```python
from build123d import *

# Parameters (mm, degrees)
F1_DEPTH       = 5
F2_W           = 15
F2_H           = 5
F3_DEPTH       = 10
F4_R           = 5
F6_D           = 4.2
F6_CSINK_D     = 8.96
F6_CSINK_ANGLE = 90


with BuildPart() as f1:
    # F0 (on Top) → F1 (new body)
    with BuildSketch(Plane.XY):
        with BuildLine():
            Line((29.5, 20), (-29.5, 20))
            ThreePointArc((-29.5, 20), (-31.62132, 19.12132), (-32.5, 17))
            Line((-32.5, 17), (-32.5, -2.5))
            ThreePointArc((-32.5, -2.5), (-31.767767, -4.267767), (-30, -5))
            ThreePointArc((-30, -5), (-28.232233, -4.267767), (-27.5, -2.5))
            Line((-27.5, -2.5), (-27.5, 15))
            Line((-27.5, 15), (27.5, 15))
            Line((27.5, 15), (27.5, -15))
            Line((27.5, -15), (-27.5, -15))
            Line((-27.5, -15), (-30, -15))
            ThreePointArc((-30, -15), (-31.767767, -15.732233), (-32.5, -17.5))
            ThreePointArc((-32.5, -17.5), (-31.767767, -19.267767), (-30, -20))
            Line((-30, -20), (29.5, -20))
            ThreePointArc((29.5, -20), (31.62132, -19.12132), (32.5, -17))
            Line((32.5, -17), (32.5, 17))
            ThreePointArc((32.5, 17), (31.62132, 19.12132), (29.5, 20))
        make_face()
    extrude(amount=F1_DEPTH)

    # F2 (on face) → F3 (join)
    with BuildSketch(Plane.XY.offset(5)):
        with Locations((-14.375, -17.5)):
            Rectangle(F2_W, F2_H)
        with Locations((13.125, -17.5)):
            Rectangle(F2_W, F2_H)
    extrude(amount=F3_DEPTH)

    # F4
    f4_edges = [f1.edges().sort_by_distance(p)[0] for p in [
        (-21.875, -17.5, 15),
        (-6.875, -17.5, 15),
        (5.625, -17.5, 15),
        (20.625, -17.5, 15),
    ]]
    fillet(f4_edges, radius=F4_R)

    # F6 (through all)
    with Locations(Plane(origin=(0, -15, 0), x_dir=(-1, 0, 0), z_dir=(0, 1, 0))):
        with Locations((14.375, 10), (-14.375, 10)):
            CounterSinkHole(F6_D / 2, F6_CSINK_D / 2, counter_sink_angle=F6_CSINK_ANGLE)


solid = f1.part
```
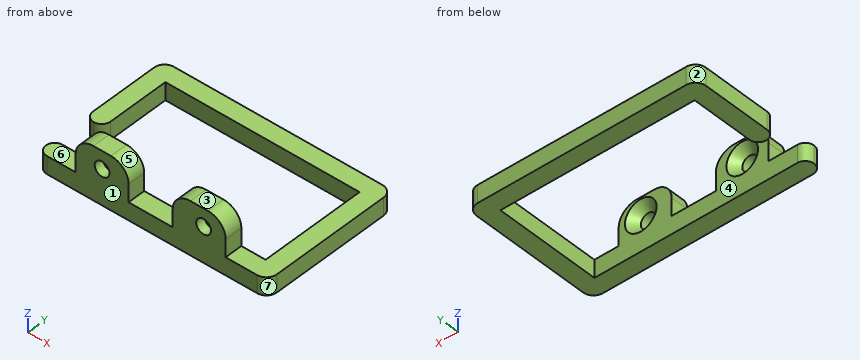
Input: part model. Units: mm. Frame: model coordinates. Face numbers are marked on the shaded views. A direction names the side the tool comes from. Round coordinates to 2 decimals unless told otherwise and drop trailing zeros. Write each loop counter-clockwise with the first axis right and the second up, starting at its lowest first coordinate (ties: lowest second). Pieces come first, ordered by that corner, then holes. Notation, with made-up numbers: M 58,32.25 L 115,32.25 A20 ccw 115,58.25 Z; hole C -26.5,62 d4. An arc over 180 degrees is marked long. Write each question's results on one line, items separated by ' | '.
Q1. Draft query along Y for the marked faces 1, 2, 3 and 4. Return one class per face: released by +Y, released by -Y, zero draft, split by the parting line, or undercut.
Results:
face 1: released by -Y | face 2: released by +Y | face 3: zero draft | face 4: undercut
Q2. Section query C-C (y = -13). Return loops of the section in (x, z).
Results:
outline: M 27.5,0 L 32.5,0 L 32.5,5 L 27.5,5 Z
Q3. Section query B-B (z = 3.25). Return loops of the section in (x, y), and give its area (3 significant figures).
Results:
outline: M -32.5,-2.5 A2.5 ccw -27.5,-2.5 L -27.5,15 L 27.5,15 L 27.5,-15 L -30,-15 A2.5 ccw -30,-20 L 29.5,-20 A3 ccw 32.5,-17 L 32.5,17 A3 ccw 29.5,20 L -29.5,20 A3 ccw -32.5,17 Z | area: 889 mm^2
Q4. Pin query (flat end, axial travel): P1, Ø4, axis at y = -17, z = 7.5, coming from the -X side (3 decimals); P2, Ø1.5, axis at x = -24.5, y = -17, coming from the +Z side; P3, Ø1.5, axis at y = -18, z = 7, coming from the +X side (3 decimals). Return the tip coordinate at first contact, or that it passes through.
Results:
P1: stops at x = -21.875 | P2: stops at z = 5 | P3: stops at x = 20.625
Q5. Section query A-A (y = 8). Return loops of the section in (x, z), and give its area (3 significant figures).
Results:
outline: M -32.5,0 L -27.5,0 L -27.5,5 L -32.5,5 Z; M 27.5,0 L 32.5,0 L 32.5,5 L 27.5,5 Z | area: 50.0 mm^2
Q6. Line query: line 1 along X through (y, z) = (-18.8, 10) (3 decimals); line 2 along Y through (x, z) = (-6, 1.25); line 3 along Y through (x, z) = (14.5, 5.25). Output: solid intervals per line, ascending.
Results:
line 1: x = -21.875 to -16.475, -12.275 to -6.875, 5.625 to 12.275, 16.475 to 20.625 | line 2: y = -20 to -15, 15 to 20 | line 3: y = -20 to -15
Q7. Access query for the marked faces 5, 6 and 7. Directions: +Z, -Z, +X, -X, +Y, -Y. A direction counts if a zero-diameter tool reaches every point of the face in a straight line with its end or side. Return the directions, or none.
Results:
face 5: +Z, +Y, -Y | face 6: +Z, -X, +Y, -Y | face 7: +Z, -Z, +X, -Y
